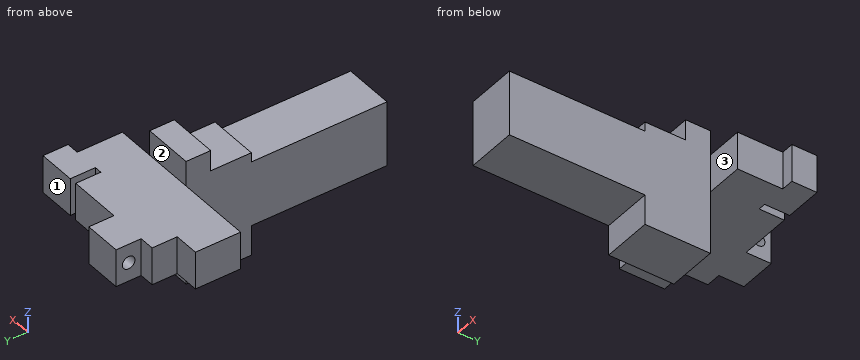
Autodesk Inventor part; units mm, degrees
ref_plane "YZ Plane" through (0, 0, 0) normal (1, 0, 0) x (0, 1, 0)
ref_plane "XZ Plane" through (0, 0, 0) normal (0, 1, 0) x (-1, 0, 0)
ref_plane "XY Plane" through (0, 0, 0) normal (0, 0, 1) x (1, 0, 0)
sketch "Sketch4" plane through (0, 0, 0) normal (0, 0, 1) x (1, 0, 0)
  line L0 (0, 0) -> (20, 0)
  line L1 (20, 0) -> (20, 54)
  line L2 (20, 54) -> (0, 54)
  line L3 (0, 54) -> (0, 0)
  dimension "d18" = 20
  dimension "d19" = 54
extrude "Extrusion4" add sketch "Sketch4" along normal mid plane 26
sketch "Sketch5" plane through (0, 54, 13) normal (0, 1, 0) x (1, 0, 0)
  line L0 (0, -12) -> (20, -12)
  line L1 (20, -12) -> (20, 38)
  line L2 (20, 38) -> (0, 38)
  line L3 (0, 38) -> (0, -12)
  line L4 (20, 26) -> (20, 0)
  line L5 (0, 26) -> (0, 0)
  point P0 (0, 13)
  point P1 (10, 38)
  point P2 (0, 13)
  dimension "d22" = 20
  dimension "d23" = 50
  dimension "d24" = 25
extrude "Extrusion5" add sketch "Sketch5" along normal blind 26
sketch "Sketch6" plane through (0, 0, 0) normal (0, 0, 1) x (1, 0, 0)
  line L0 (35, 80) -> (-30, 80)
  line L1 (-30, 80) -> (-30, 98)
  line L2 (-30, 98) -> (35, 98)
  line L3 (35, 98) -> (35, 80)
  line L4 (0, 80) -> (20, 80)
  line L5 (20, 54) -> (20, 80)
  line L6 (0, 54) -> (0, 80)
  line L7 (-20, 98) -> (22, 98)
  line L8 (22, 98) -> (22, 108)
  line L9 (22, 108) -> (-20, 108)
  line L10 (-20, 108) -> (-20, 98)
  line L11 (25, 98) -> (40, 98)
  line L12 (40, 98) -> (40, 108)
  line L13 (40, 108) -> (25, 108)
  line L14 (25, 108) -> (25, 98)
  line L15 (-14, 108) -> (1, 108)
  line L16 (1, 108) -> (1, 118)
  line L17 (1, 118) -> (-14, 118)
  line L18 (-14, 118) -> (-14, 108)
  point P0 (0, 0)
  point P1 (35, 98)
  point P2 (22, 98)
  point P3 (-20, 103)
  point P4 (-14, 113)
  dimension "d27" = 18
  dimension "d28" = 15
  dimension "d29" = 30
  dimension "d32" = 10
  dimension "d33" = 10
  dimension "d34" = 15
  dimension "d38" = 3
  dimension "d39" = 15
  dimension "d40" = 5
  dimension "d41" = 10
  dimension "d42" = 6
extrude "Extrusion6" add sketch "Sketch6" along normal blind 15
sketch "Sketch9" plane through (0, 0, 13) normal (0, 0, 1) x (1, 0, 0)
  point P0 (0, 0)
  point P1 (10, 29.6336)
sketch "Sketch10" plane through (0, 0, 15) normal (0, 0, 1) x (1, 0, 0)
  point P0 (0, 0)
  point P1 (-8.9634, 87.1554)
sketch "Sketch11" plane through (40, 98, 15) normal (1, 0, 0) x (0, 0, -1)
  point P0 (15, -98)
  point P1 (7.5, 5)
sketch "Sketch12" plane through (20, 0, 13) normal (1, 0, 0) x (0, 0, -1)
  point P0 (13, 0)
  point P1 (13, 63.2643)
sketch "Sketch13" plane through (-14, 108, 15) normal (-1, 0, 0) x (0, 0, 1)
  circle A0 centre (-7.5, 5) radius 2.5
  line L0 (-15, 10) -> (0, 10)
  line L1 (0, -10) -> (0, 0)
  line L2 (-15, 10) -> (0, 0) construction
  point P0 (-15, -108)
  dimension "d35" = 5
extrude "Extrusion7" cut sketch "Sketch13" against normal through all
sketch "Sketch14" plane through (20, 0, 13) normal (1, 0, 0) x (0, 0, -1)
  line L0 (-31.824, 26.3525) -> (-3.7474, 26.3525)
  line L1 (-3.7474, 26.3525) -> (-3.7474, 70.1914)
  line L2 (-3.7474, 70.1914) -> (-31.824, 70.1914)
  line L3 (-31.824, 70.1914) -> (-31.824, 26.3525)
  line L4 (-31.824, 26.3525) -> (-3.7474, 70.1914) construction
  line L5 (-3.7474, 26.3525) -> (-31.824, 70.1914) construction
  point P0 (13, 0)
  point P1 (-17.7857, 48.272)
extrude "Extrusion8" cut sketch "Sketch14" against normal through all
properties part number "micromanipulator"
Check sheet for the modelled part. Datum: model origin and axes. Units: mm. Face numbers are marked on the shaded views. A direction names the side the tool comes from. Round coordinates to 2 decimals unless told otherwise and drop trailing zeros. Loops run counter-clockwise (first coordinate to the right, second up) from the corner with the lowest first, then second, coordinate; pieces in that order, holes last.
1. Scan lines: probe 1 along Y at (x, z) = (-3.25, 7.5); probe 2 along X at (y, z) = (85.5, 3); probe 3 along X at (y, z) = (74, 18.5). Record each from-to range of solid material in increasing order.
2. Set-up check for the marked faces 1, 2 and 3: record each of +Z, -Z, +X, -X, +Y, -Y from which the full face is reachable in a straight line by a thin tool's end or side.
3. Gauge pin test, flat ends, axial feed: pin 1 Ø1.5 at (y, z) = (68, -5.5) entering from +X; pin 2 Ø8 at (x, z) = (27.5, 8) entering from -Y; pin 3 Ø3 at (y, z) = (103, 8.5) entering from -X; pin 4 Ø4 at (x, z) = (21, 0) entering from -Y. Record the tip position at first contact, or that the pin passes through.
4. Sectioned sample at D-D on z = -9. Record the boundary of the cut face in (x, y).
5. Sectioned sample at B-B on z = 7.5. Record the boundary of the cut face in (x, y), and give its area (4 significant figures).
6. Sectioned sample at A-A on y = 113. Record the boundary of the cut face in (x, z), and give its area (3 significant figures).
7. Sectioned sample at C-C on y = 61. Record the boundary of the cut face in (x, z).
Recorded:
1. probe 1: y = 80 to 110.5, 115.5 to 118
1. probe 2: x = -30 to 35
1. probe 3: x = 0 to 20
2. face 1: +Z, -Z, +X, +Y
2. face 2: +Z, +X, -X, +Y
2. face 3: +Z, -Z, +X, -Y
3. pin 1: stops at x = 20
3. pin 2: stops at y = 80
3. pin 3: stops at x = -20
3. pin 4: stops at y = 0
4. outline: (0, 0) - (20, 0) - (20, 80) - (0, 80) - close
5. outline: (-30, 80) - (0, 80) - (0, 0) - (20, 0) - (20, 80) - (35, 80) - (35, 98) - (40, 98) - (40, 108) - (25, 108) - (25, 98) - (22, 98) - (22, 108) - (1, 108) - (1, 110.5) - (-14, 110.5) - (-14, 108) - (-20, 108) - (-20, 98) - (-30, 98) - close; (-14, 115.5) - (1, 115.5) - (1, 118) - (-14, 118) - close
5. area: 3,415 mm2
6. outline: (-14, 0) - (1, 0) - (1, 5) - (-14, 5) - close; (-14, 10) - (1, 10) - (1, 15) - (-14, 15) - close
6. area: 150 mm2
7. outline: (0, -25) - (20, -25) - (20, 16.75) - (0, 16.75) - close
